Verification items for this drawing (mm, ordinates from the low corner). A direction names the side the tool comes from. Give positions to 0.01 mm unless a question says otherwise; leave off trailing zeros. Loops run counter-clockwise (first coordinate to the right, second up) from the corner with the lowest first, then second, coordinate; pieces in that order, holes last. Notation, with made-up numbers: (11.5, 32) -> (35.5, 32) arc R28 cw to (35.5, 69) -> close; hole circle Ø5 at (54.25, 73.25). An arc over 180 degrees is marked (long way). Answer in a Markdown table with one row per item. Add a question column.
Q1. Release check for a two-part mould opening along X. For the marked faces 1, 2 and 3 record: pulls with the +X half, pulls with the -X half, needs draft (parallel to the pull), parting line crosses it, or undercut.
Q2. Set-up check for the marked faces 4, 5 and 6: record each of +Z, -Z, +X, -X, +Y, -Y from which the full face is reachable in a straight line by a thin tool's end or side.
Q3. Section check A-A on y = 0.35. Enter the section's corners in (x, z).
Q4. Section check D-D on y = 2.15. Enter the section's corners in (x, z), and give its area (3 significant figures).
Q5. Section check C-C on z = 4.75. Enter the section's corners in (x, y).
Q6. Gauge pin test, flat ends, axial feed: P1, Ø1.5, axis at y = 3, z = 8, coming from the +X side; P2, Ø1.6, axis at x = 8.5, z = 5.5, coming from the +Y side; P3, Ø6, axis at x = 9, z = 4.5, coming from the +Y side; P4, Ø0.5, axis at x = 2.5, z = 4.5, coming from the -Y side. Record the tip position at first contact, or that the pin passes through.
Q7. Material ranges on probe 1 along X at (y, z) = (0.6, 5.5); probe 2 along X at (y, z) = (2.8, 5); probe 3 along Z at (x, y) = (8.5, 0.85), recorded low to high.
Q8. Section check B-B on x = 8.5. Enter the section's corners in (y, z), and give its area (3 significant figures).
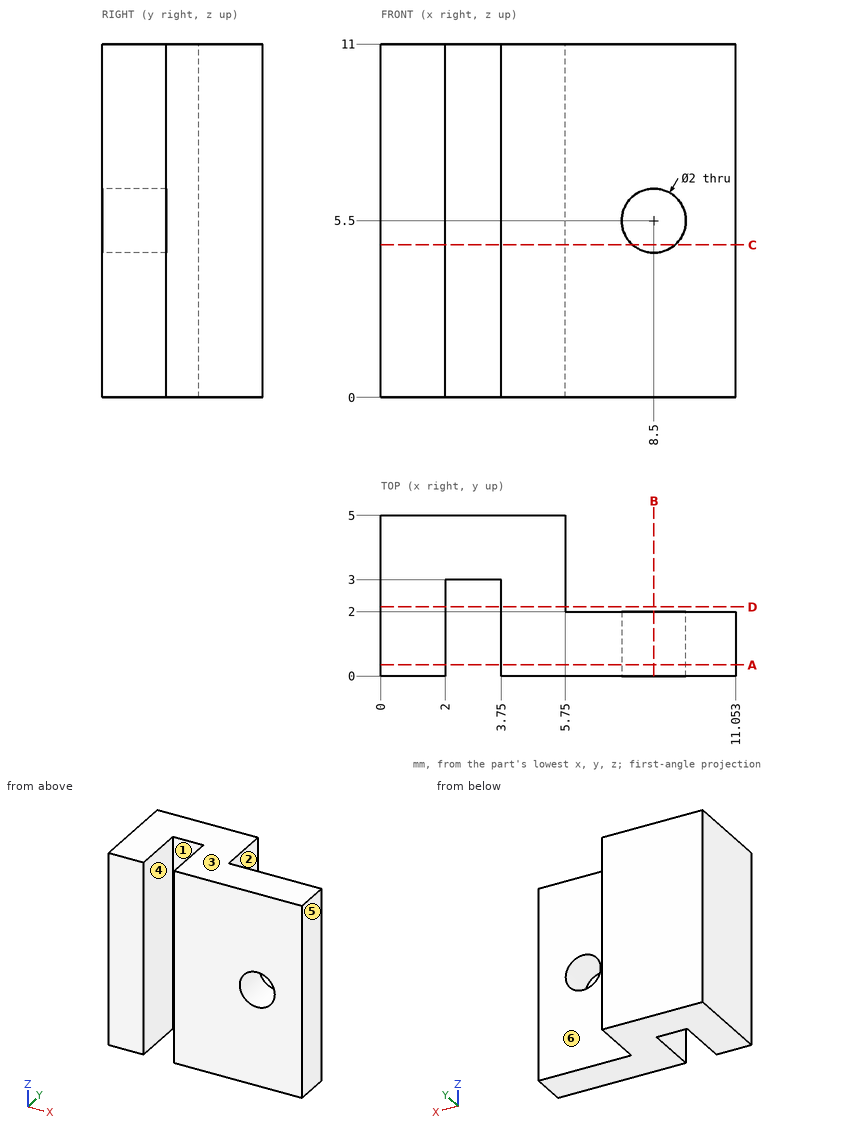
Taken from the geometry:
| question | item | result |
|---|---|---|
| 1 | face 1 | undercut |
| 1 | face 2 | pulls with the +X half |
| 1 | face 3 | needs draft |
| 2 | face 4 | +Z, -Z, -Y |
| 2 | face 5 | +Z, -Z, +X, +Y, -Y |
| 2 | face 6 | +Z, -Z, +X, +Y |
| 3 | outline | (0, 0) -> (2, 0) -> (2, 11) -> (0, 11) -> close; (3.75, 0) -> (11.05, 0) -> (11.05, 11) -> (3.75, 11) -> close; hole circle Ø2 at (8.5, 5.5) |
| 4 | outline | (0, 0) -> (2, 0) -> (2, 11) -> (0, 11) -> close; (3.75, 0) -> (5.75, 0) -> (5.75, 11) -> (3.75, 11) -> close |
| 4 | area | 44.0 mm² |
| 5 | outline | (0, 0) -> (2, 0) -> (2, 3) -> (3.75, 3) -> (3.75, 0) -> (7.84, 0) -> (7.84, 2) -> (5.75, 2) -> (5.75, 5) -> (0, 5) -> close; (9.16, 0) -> (11.05, 0) -> (11.05, 2) -> (9.16, 2) -> close |
| 6 | P1 | stops at x = 5.75 |
| 6 | P2 | passes through |
| 6 | P3 | stops at y = 2 |
| 6 | P4 | stops at y = 3 |
| 7 | probe 1 | x = 0 to 2, 3.75 to 7.5, 9.5 to 11.05 |
| 7 | probe 2 | x = 0 to 2, 3.75 to 5.75 |
| 7 | probe 3 | z = 0 to 4.5, 6.5 to 11 |
| 8 | outline | (0, 0) -> (2, 0) -> (2, 4.5) -> (0, 4.5) -> close; (0, 6.5) -> (2, 6.5) -> (2, 11) -> (0, 11) -> close |
| 8 | area | 18.0 mm² |
